Job drawing, mm, ordinate dimensions from the low corner. One solid piece. A direction names the side the tool comes from. Give positions to 0.01 mm unless a question says otherwise; leave off trailing zeros. Write each loop counter-clockwise with the first axis right and the second up, starting at its lowest first coordinate (ties: lowest second). Pieces come first, ordered by that corner, then holes. Notation, with made-up numbers: (77.25, 16.5) -> (82.25, 16.5) arc R23 ccw to (82.25, 50.5) -> close; hole circle Ø11 at (65, 52). An arc over 180 degrees is marked (long way). One line per question, with ' | ' between items. Start each with the question number.
(1) Drill centre lines: probe 1 along X at (y, z) = (3, 3.25); probe 2 along Y at (x, z) = (1.25, 4.5); probe 3 along Y at (x, z) = (4.5, 2.25) (1 decimal). Where is each one in solid material? Low to high. Write a range as from..to.
(2) Tool access for the marked faces 4 and 5: list every direction of +Z, -Z, +X, -X, +Y, -Y with a clear straight run to the whole face (end or side of a thin tool).
(3) Band-saw the part on A-A, the plane z = 4. Give the cut face in (x, y).
(4) Band-saw the part on B-B, the plane x = 5.25. Give the cut face in (y, z), and give its area (3 significant figures).
(5) Pin check, flat tips, straight feed: P1, Ø1, axis at x = 10, y = 3, coming from the -Z side; P2, Ø0.8, axis at y = 3.5, z = 4.5, coming from the -X side; P3, Ø1.2, axis at x = 1, z = 4, coming from the +Y side. Stop position of each tip, or through.
(6) Pull direction Z, two halves, no side cores. Call the marked faces 1, 2 and 3: released by +Z, released by -Z, zero draft, split by the parting line, or undercut.
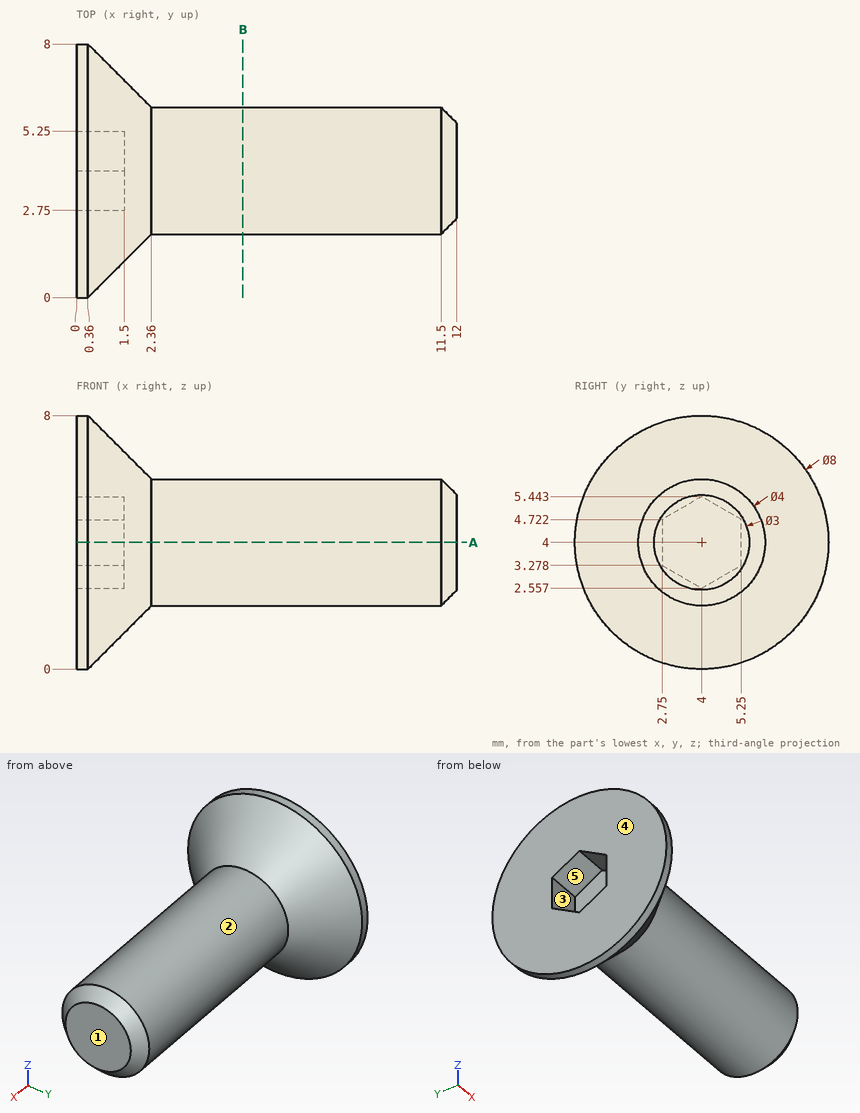
Results:
1) probe 1: x = 1.5..12 | probe 2: y = 0.93..2.75, 5.25..7.07 | probe 3: y = 3..5
2) face 4: +Z, -Z, -X, +Y, -Y | face 5: -X
3) outline: (0, 0) -> (0.36, 0) -> (2.36, 2) -> (11.5, 2) -> (12, 2.5) -> (12, 5.5) -> (11.5, 6) -> (2.36, 6) -> (0.36, 8) -> (0, 8) -> (0, 5.25) -> (1.5, 5.25) -> (1.5, 2.75) -> (0, 2.75) -> close
4) outline: circle Ø4 at (4, 4) | area: 12.6 mm²
5) P1: stops at z = 2.06 | P2: stops at x = 1.5 | P3: stops at y = 7.96
6) face 1: zero draft | face 2: split by the parting line | face 3: undercut
